The listing builds one solid part. Answer for the finished solid, in the listing's coordinates (mm). A direction names the side the tool comes from. Give positions to 0.01 mm unless a question says otherwise; leave off trailing zeros. Loops run counter-clockwise (first coordinate to the right, second up) from the corner with the lowest first, then second, coordinate; pieces in that order, holes last.
Item 1: The mould has two halves that part along Y. Classify faces 6 (the face through (-0.16, 13.24, 0.51)), 7 (the face through (-13.507, 0.867, -2.405)), 8 (the face through (-3, -12, 1.5)), 9 (the face through (-6.5, -8, 1)): pulls with the +Y half, pulls with the -Y half, needs draft (parallel to the pull), parting line crosses it, or undercut.
Item 2: Each of these flat-tipped pins is pushed along its axis until it touches: pin 1 Ø3 at (x, y) = (0, -12) entering from -Z; pin 2 Ø1.9 at (y, z) = (0.5, 3.5) entering from +X; pin 3 Ø2 at (x, z) = (2, 1.5) entering from -Y. Where does it stop, or does it pass through?
Item 3: A tool of negligible diameter and unlimited length cuts with its end or side. For faces 1 (the face through (5, 0, 3)), 2 (the face through (-2, 7, 1.5)), 3 (the face through (-3, 12, 1.5)), 4 (the face through (-5.5, 0, -1)), 5 (the face through (-2, -16.2, 1.5)), from which of +Z, -Z, +X, -X, +Y, -Y can it reach the whole face along a straight path? Write none if from no direction.
Item 4: Section D-D, the plane y = 7 is taken. Give the vertices of the cut face in (x, z), and give its area (3 significant figures).
Item 5: Section B-B, the plane z = -1.5 is taken. Give the vertices of the cut face in (x, y), and give its area (3 significant figures).
Item 6: Section C-C, the plane x = -10.5 is taken. Give the vertices of the cut face in (y, z), and give its area (3 significant figures).
Item 7: Consider line 1 along Y through (x, z) = (-4.25, 3); line 2 along X through (y, z) = (-2, 2.5); line 3 along Y through (x, z) = (-11, 1.5). Determine where each line is inside the solid, lowest interval first.
Item 8: Section A-A, the plane y = 0 is taken. Give the vertices of the cut face in (x, z).
from build123d import *

# Parameters (mm, degrees)
F1_DEPTH  = 2
F2_W      = 4
F2_H      = 40.789261
F3_DEPTH  = 1
F5_R      = 4.25
F6_DEPTH  = 19
F7_R      = 4.394544
F7_R_2    = 4.25
F7_R_3    = 4
F8_DEPTH  = 1
F9_W      = 12
F9_H      = 12.99651
F10_DEPTH = 25
F11_R     = 3
F12_DEPTH = 1
F13_R     = 1.25
F14_DEPTH = 3.751
F15_R     = 1.25
F16_DEPTH = 3.751


with BuildPart() as f1:
    # F0 (on Top) → F1 (new body)
    with BuildSketch(Plane.XY):
        with BuildLine():
            ThreePointArc((0, 18.5), (-4.596194, 16.596194), (-6.5, 12))
            Line((-6.5, 12), (-6.5, -12))
            ThreePointArc((-6.5, -12), (-4.596194, -16.596194), (0, -18.5))
            ThreePointArc((0, -18.5), (4.596194, -16.596194), (6.5, -12))
            Line((6.5, -12), (6.5, 12))
            ThreePointArc((6.5, 12), (4.596194, 16.596194), (0, 18.5))
        make_face()
    extrude(amount=F1_DEPTH)

    # F2 (on face) → F3 (cut)
    with BuildSketch(Plane.XY.offset(2)):
        with Locations((0, 0.259061)):
            Rectangle(F2_W, F2_H)
    extrude(amount=-F3_DEPTH, mode=Mode.SUBTRACT)

    # F5 (on offset) → F6 (join)
    with BuildSketch(Plane.YZ.offset(-14)):
        with Locations((0, 1.5)):
            Circle(F5_R)
    extrude(amount=F6_DEPTH)

    # F7 (on face) → F8 (cut)
    with BuildSketch(Plane(origin=(-14, 0, 0), x_dir=(0, -1, 0), z_dir=(-1, 0, 0))):
        with Locations((0, 1.5)):
            Circle(F7_R)
        with Locations((0, 1.5)):
            Circle(F7_R_2, mode=Mode.SUBTRACT)
        with Locations((0, 1.5)):
            Circle(F7_R_2)
        with Locations((0, 1.5)):
            Circle(F7_R_3, mode=Mode.SUBTRACT)
    extrude(amount=-F8_DEPTH, mode=Mode.SUBTRACT)

    # F9 (on face) → F10 (cut)
    with BuildSketch(Plane(origin=(0, 0, 0), x_dir=(1, 0, 0), z_dir=(0, 0, -1))):
        with Locations((0.5, -0.554225)):
            Rectangle(F9_W, F9_H)
    extrude(amount=F10_DEPTH, mode=Mode.SUBTRACT)

    # F11 (on face) → F12 (cut, through all)
    with BuildSketch(Plane.XY.offset(1)):
        with Locations((0, -12)):
            Circle(F11_R)
        with Locations((0, 12)):
            Circle(F11_R)
    extrude(amount=F12_DEPTH, mode=Mode.SUBTRACT)

    # F13 (on face) → F14 (cut, through all)
    with BuildSketch(Plane.XY.offset(1)):
        with Locations((0, -12)):
            Circle(F13_R)
    extrude(amount=-F14_DEPTH, mode=Mode.SUBTRACT)

    # F15 (on face) → F16 (cut, through all)
    with BuildSketch(Plane.XY.offset(1)):
        with Locations((0, 12)):
            Circle(F15_R)
    extrude(amount=-F16_DEPTH, mode=Mode.SUBTRACT)


solid = f1.part
Worked answers:
1. face 6: undercut
1. face 7: parting line crosses it
1. face 8: undercut
1. face 9: needs draft
2. pin 1: stops at z = 0
2. pin 2: stops at x = 5
2. pin 3: stops at y = -18.4
3. face 1: +Z, +X, +Y, -Y
3. face 2: +Z, +Y
3. face 3: +Z
3. face 4: -Z, +X, +Y, -Y
3. face 5: +Z, -Y
4. outline: (-6.5, 0) - (6.5, 0) - (6.5, 2) - (2, 2) - (2, 1) - (-2, 1) - (-2, 2) - (-6.5, 2) - close
4. area: 22.0 mm2
5. outline: (-14, -2.65) - (-13, -2.65) - (-13, -3.01) - (-5.5, -3.01) - (-5.5, 3.01) - (-13, 3.01) - (-13, 2.65) - (-14, 2.65) - close
5. area: 50.4 mm2
6. outline: circle Ø8.5 at (0, 1.5)
6. area: 56.7 mm2
7. line 1: y = -3.98 to 3.98
7. line 2: x = -14 to 5
7. line 3: y = -4.25 to 4.25
8. outline: (-14, -2.5) - (-13, -2.5) - (-13, -2.75) - (-5.5, -2.75) - (-5.5, 0) - (6.5, 0) - (6.5, 2) - (5, 2) - (5, 5.75) - (-13, 5.75) - (-13, 5.5) - (-14, 5.5) - close
